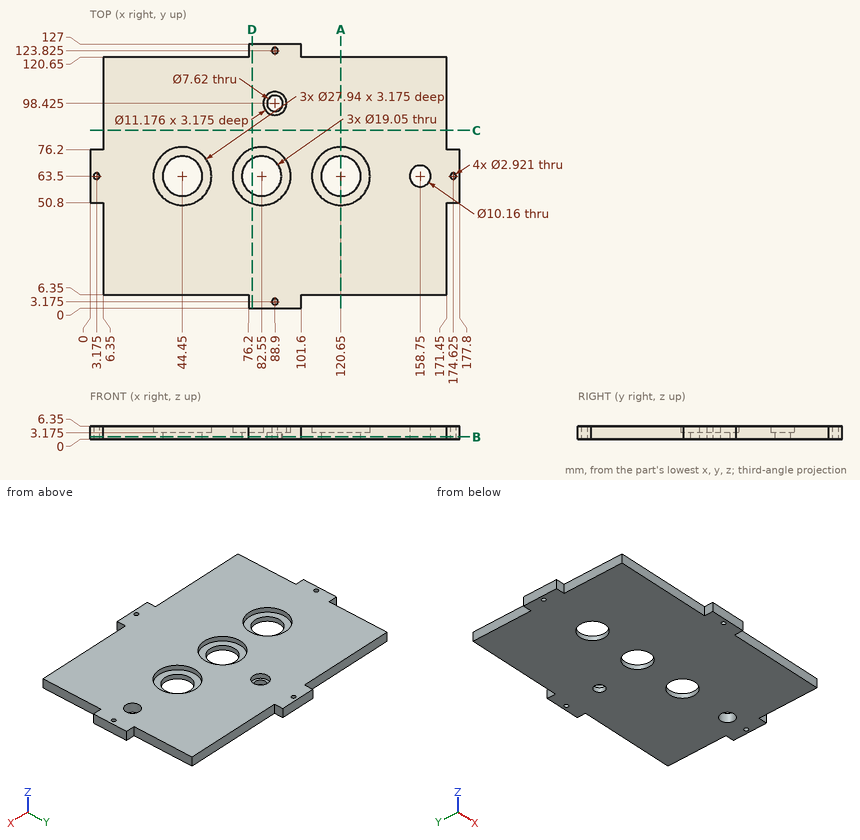
Here's the drawing with two shaded views (mm, measured from the low corner). I have some questions. Round coordinates to 2 decimals unless told otherwise and drop trailing zeros. Write each loop counter-clockwise with the first axis right and the second up, starting at its lowest first coordinate (ties: lowest second). Pieces come first, ordered by that corner, then holes. Notation, with made-up numbers: M -11.75,0.5 L 8.25,0.5 A25 ccw 8.25,25.5 Z; hole C 76,87.25 d4. An arc over 180 degrees is marked long. Answer in a Markdown table with one row per item. Add a question column.
Q1. Imagine slicing it at A-A (x = 120.65). Please give me the cut outline in (y, z) (3 decimals).
Q2. Imagine slicing it at D-D (x = 78). Please give me the cut outline in (y, z) (3 decimals), then the cut area to 3 significant figures.
Q3. Imagine slicing it at C-C (y = 85.5). Please give me the cut outline in (x, z), then the cut area to 3 significant figures.
Q4. If I drill on line 1 (Y direction, x = 88.9, z = 4.15); line 2 (X direction, y = 52, z = 5); line 3 (X direction, y = 69.5, z = 4.25), over which ranges is the centre line in solid material (lowest first)? Write a range as from..to.
Q5. Will these pins go through, and if not, where does the flat tip stop? pin 1 Ø1 at (y, z) = (37, 2.5) entering from +X; pin 2 Ø1.5 at (y, z) = (106, 5.5) entering from -X; pin 3 Ø1.5 at (x, z) = (141.5, 1) entering from -Y.
Q6. Imagine slicing it at B-B (z = 1.25). Give the number of separate pieces and of enclosed holes in the cut face, then the cut area to 3 significant figures.
Values:
| question | item | result |
|---|---|---|
| 1 | outline | M 6.35,0 L 53.975,0 L 53.975,3.175 L 49.53,3.175 L 49.53,6.35 L 6.35,6.35 Z; M 73.025,0 L 120.65,0 L 120.65,6.35 L 77.47,6.35 L 77.47,3.175 L 73.025,3.175 Z |
| 2 | outline | M 0,0 L 55.132,0 L 55.132,3.175 L 50.292,3.175 L 50.292,6.35 L 0,6.35 Z; M 71.868,0 L 127,0 L 127,6.35 L 76.708,6.35 L 76.708,3.175 L 71.868,3.175 Z |
| 2 | area | 669 mm^2 |
| 3 | outline | M 6.35,0 L 171.45,0 L 171.45,6.35 L 6.35,6.35 Z |
| 3 | area | 1,050 mm^2 |
| 4 | line 1 | 0..1.71, 4.64..51.06, 75.94..92.84, 104.01..122.36, 125.29..127 |
| 4 | line 2 | 0..36.52, 52.38..74.62, 90.48..112.72, 128.58..177.8 |
| 4 | line 3 | 0..31.83, 57.07..69.93, 95.17..108.03, 133.27..177.8 |
| 5 | pin 1 | x = 171.45 |
| 5 | pin 2 | x = 6.35 |
| 5 | pin 3 | y = 6.35 |
| 6 | separate pieces | 1 |
| 6 | enclosed holes | 9 |
| 6 | area | 18,500 mm^2 |
